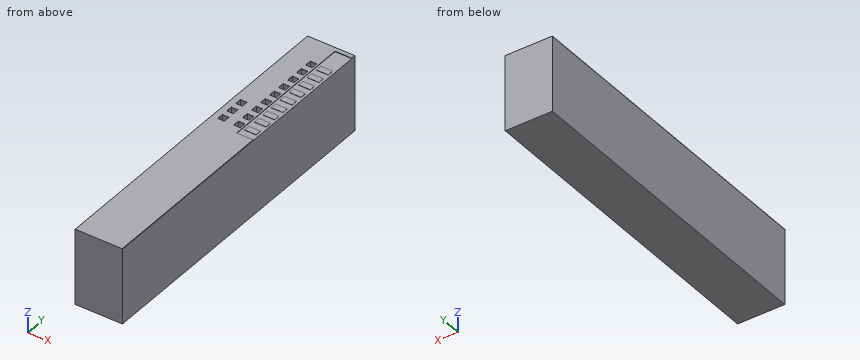
from build123d import *

# Parameters (mm, degrees)
CROQUIS1_W              = 178.587886288
CROQUIS1_H              = 1245.447721363
CROQUIS1_W_2            = 25
CROQUIS1_H_2            = 25
SALIENTE_EXTRUIR2_DEPTH = 285
CROQUIS2_W              = 178.587886288
CROQUIS2_H              = 552.844893509
SALIENTE_EXTRUIR3_DEPTH = 1
CROQUIS5_W              = 25
CROQUIS5_H              = 25
SALIENTE_EXTRUIR4_DEPTH = 2
CROQUIS10_W             = 44.39506519
CROQUIS10_H             = 23.654322964
CROQUIS10_H_2           = 23.654322963
SALIENTE_EXTRUIR5_DEPTH = 1


with BuildPart() as part:
    # Croquis1 → Saliente-Extruir2 (new body)
    with BuildSketch(Plane.XY):
        with Locations((121.784181129, -381.025603562)):
            Rectangle(CROQUIS1_W, CROQUIS1_H)
        with Locations((174.990237985, -163.957841157)):
            Rectangle(CROQUIS1_W_2, CROQUIS1_H_2, mode=Mode.SUBTRACT)
        with Locations((115.437079382, 126.027179256)):
            Rectangle(CROQUIS1_W_2, CROQUIS1_H_2, mode=Mode.SUBTRACT)
        with Locations((115.437079382, 77.694179256)):
            Rectangle(CROQUIS1_W_2, CROQUIS1_H_2, mode=Mode.SUBTRACT)
        with Locations((115.437079382, 29.364179256)):
            Rectangle(CROQUIS1_W_2, CROQUIS1_H_2, mode=Mode.SUBTRACT)
        with Locations((115.437079382, -18.965820744)):
            Rectangle(CROQUIS1_W_2, CROQUIS1_H_2, mode=Mode.SUBTRACT)
        with Locations((114.990237985, -67.291541157)):
            Rectangle(CROQUIS1_W_2, CROQUIS1_H_2, mode=Mode.SUBTRACT)
        with Locations((114.990237985, -115.624841157)):
            Rectangle(CROQUIS1_W_2, CROQUIS1_H_2, mode=Mode.SUBTRACT)
        with Locations((114.990237985, -163.957841157)):
            Rectangle(CROQUIS1_W_2, CROQUIS1_H_2, mode=Mode.SUBTRACT)
        with Locations((114.990237985, -212.287841157)):
            Rectangle(CROQUIS1_W_2, CROQUIS1_H_2, mode=Mode.SUBTRACT)
        with Locations((114.990237985, -260.617841157)):
            Rectangle(CROQUIS1_W_2, CROQUIS1_H_2, mode=Mode.SUBTRACT)
        with Locations((174.990237985, -212.287841157)):
            Rectangle(CROQUIS1_W_2, CROQUIS1_H_2, mode=Mode.SUBTRACT)
        with Locations((174.990237985, -260.617841157)):
            Rectangle(CROQUIS1_W_2, CROQUIS1_H_2, mode=Mode.SUBTRACT)
    extrude(amount=-SALIENTE_EXTRUIR2_DEPTH)

    # Croquis2 → Saliente-Extruir3 (add)
    with BuildSketch(Plane(origin=(0, 0, -285), x_dir=(-1, 0, 0), z_dir=(0, 0, -1))):
        with Locations((-121.784181129, -34.724189635)):
            Rectangle(CROQUIS2_W, CROQUIS2_H)
    extrude(amount=-SALIENTE_EXTRUIR3_DEPTH)

    # Croquis5 → Saliente-Extruir4 (add)
    with BuildSketch(Plane.XY):
        Polygon((40.133927115, 241.69825712), (187.776914698, 241.69825712), (211.134564186, 241.69825712), (211.134564186, -1003.749464243), (33.378525324, -1003.749464243), (33.378525324, -301.90284108), (95.791395616, -301.90284108), (95.791395616, 225.342265798), (32.490237985, 225.342265798), (32.490237985, 241.69825712), align=None)
        with Locations((175.276914698, -164.067102515)):
            Rectangle(CROQUIS5_W, CROQUIS5_H, mode=Mode.SUBTRACT)
        with Locations((115.723756094, 125.917917897)):
            Rectangle(CROQUIS5_W, CROQUIS5_H, mode=Mode.SUBTRACT)
        with Locations((115.723756094, 77.584917897)):
            Rectangle(CROQUIS5_W, CROQUIS5_H, mode=Mode.SUBTRACT)
        with Locations((115.723756094, 29.254917897)):
            Rectangle(CROQUIS5_W, CROQUIS5_H, mode=Mode.SUBTRACT)
        with Locations((115.723756094, -19.075082103)):
            Rectangle(CROQUIS5_W, CROQUIS5_H, mode=Mode.SUBTRACT)
        with Locations((115.276914698, -67.400802515)):
            Rectangle(CROQUIS5_W, CROQUIS5_H, mode=Mode.SUBTRACT)
        with Locations((115.276914698, -115.734102515)):
            Rectangle(CROQUIS5_W, CROQUIS5_H, mode=Mode.SUBTRACT)
        with Locations((115.276914698, -164.067102515)):
            Rectangle(CROQUIS5_W, CROQUIS5_H, mode=Mode.SUBTRACT)
        with Locations((115.276914698, -212.397102515)):
            Rectangle(CROQUIS5_W, CROQUIS5_H, mode=Mode.SUBTRACT)
        with Locations((115.276914698, -260.727102515)):
            Rectangle(CROQUIS5_W, CROQUIS5_H, mode=Mode.SUBTRACT)
        with Locations((175.276914698, -212.397102515)):
            Rectangle(CROQUIS5_W, CROQUIS5_H, mode=Mode.SUBTRACT)
        with Locations((175.276914698, -260.727102515)):
            Rectangle(CROQUIS5_W, CROQUIS5_H, mode=Mode.SUBTRACT)
    extrude(amount=SALIENTE_EXTRUIR4_DEPTH)

    # Croquis10 → Saliente-Extruir5 (add)
    with BuildSketch(Plane.XY):
        with Locations((64.427271282, 75.386790193)):
            Rectangle(CROQUIS10_W, CROQUIS10_H)
        with Locations((64.427271282, -20.708896845)):
            Rectangle(CROQUIS10_W, CROQUIS10_H_2)
        with Locations((64.427271282, -69.495937956)):
            Rectangle(CROQUIS10_W, CROQUIS10_H_2)
        with Locations((64.427271282, -118.282979068)):
            Rectangle(CROQUIS10_W, CROQUIS10_H_2)
        with Locations((62.948876097, -164.113229809)):
            Rectangle(CROQUIS10_W, CROQUIS10_H_2)
        with Locations((62.948876097, -209.94348055)):
            Rectangle(CROQUIS10_W, CROQUIS10_H_2)
        with Locations((64.427271282, 28.078144267)):
            Rectangle(CROQUIS10_W, CROQUIS10_H_2)
        with Locations((64.427271282, 124.173831305)):
            Rectangle(CROQUIS10_W, CROQUIS10_H_2)
        with Locations((64.427271282, -261.687312031)):
            Rectangle(CROQUIS10_W, CROQUIS10_H)
    extrude(amount=SALIENTE_EXTRUIR5_DEPTH)


with BuildPart() as body_2:
    # Simetría1: mirrored copy
    add(part.part.mirror(Plane(origin=(311.078124273, 0, 0), x_dir=(0, 0, 1), z_dir=(1, 0, 0))))


solid = body_2.part
CAD build for the part. Positions are in the model's coordinates, mm. Round coordinates to 2 decimals unless told otherwise and drop trailing zeros. Write item = value, one per line. Start each with the question number.
(1) Pin check, flat tips, straight feed: P1, Ø0.6, axis at y = 74.5, z = 0.5, coming from the +X side; P2, Ø4, axis at y = -27.5, z = -201.5, coming from the -X side. Stop position of each tip, or through.
(2) Probe line 1 (Y direction, x = 437, z = -235); line 2 (X direction, y = -155, z = -271.5); line 3 (X direction, y = 81, z = -84.5). List the from-to ranges inside material, lowest first. Write a range as [from, to].
(3) Cut at A-A, the plane z = -193. State how many separate pieces and enclosed holes the cut face has, then the cut area to 3 significant figures.
Model answer:
q1.P1 = 579.93
q1.P2 = 411.08
q2.line_1 = [-1003.75, -273.12], [-248.12, -224.79], [-199.79, -176.46], [-151.46, 241.7]
q2.line_2 = [411.08, 434.67], [459.67, 494.67], [519.67, 589.67]
q2.line_3 = [411.08, 494.22], [519.22, 589.67]
q3.separate_pieces = 1
q3.enclosed_holes = 12
q3.area = 215,000 mm2
